Read the model definition and answer for the solid it produces. Units are mm, in the model's axes. A direction names the side the tool comes from. Give positions to 0.01 mm unless a question says otherwise; leave off trailing zeros. Write each loop counter-clockwise with the first axis right and the second up, starting at its lowest first coordinate (ties: lowest second). Pieces come first, ordered by that corner, then holes. Notation, with made-up numbers: M 41.25,73 L 93.25,73 A32 cw 93.25,110 Z; hole C -23.5,-1 d3. An arc over 180 degrees is marked long. Put each result on its own line as item: value.
from build123d import *

# Parameters (mm, degrees)
SKETCH_1_W          = 87.4
SKETCH_1_H          = 58
EXTRUDE_1_DEPTH     = 2
EXTRUDE_2_DEPTH     = 9
SKETCH_3_W          = 2
SKETCH_3_H          = 5
EXTRUDE_3_DEPTH     = 28
SKETCH_4_W          = 28
SKETCH_4_H          = 3
EXTRUDE_4_DEPTH     = 5.4
EXTRUDE_7_DEPTH     = 58
SKETCH_6_W          = 14.323261058
SKETCH_6_H          = 15
CUT_EXTRUDE_2_DEPTH = 58
SKETCH_8_W          = 87.4
SKETCH_8_H          = 14.7
CUT_EXTRUDE_3_DEPTH = 35
SKETCH_9_W          = 87.4
SKETCH_9_H          = 58
EXTRUDE_8_DEPTH     = 2
EXTRUDE_9_DEPTH     = 29
SKETCH_11_W         = 8.812157776
SKETCH_11_H         = 15
CUT_EXTRUDE_4_DEPTH = 13
SKETCH_13_W         = 87.4
SKETCH_13_H         = 0.5
CUT_EXTRUDE_6_DEPTH = 200


with BuildPart() as part:
    # 草图1 → 凸台-拉伸1 (new body)
    with BuildSketch(Plane.XY):
        Rectangle(SKETCH_1_W, SKETCH_1_H)
    extrude(amount=EXTRUDE_1_DEPTH)

    # 草图2 → 凸台-拉伸2 (add)
    with BuildSketch(Plane.XY.offset(2)):
        Polygon((-43.7, -25), (-43.7, -27), (-13.7, -27), (-13.7, 12.3), (-43.7, 12.3), (-43.7, 10.3), (-15.7, 10.3), (-15.7, -25), align=None)
    extrude(amount=EXTRUDE_2_DEPTH)

    # 草图3 → 凸台-拉伸3 (add)
    with BuildSketch(Plane.ZY.offset(15.7)):
        with Locations((10, 7.8)):
            Rectangle(SKETCH_3_W, SKETCH_3_H)
        with Locations((10, -22.5)):
            Rectangle(SKETCH_3_W, SKETCH_3_H)
    extrude(amount=EXTRUDE_3_DEPTH)

    # 草图4 → 凸台-拉伸4 (add)
    with BuildSketch(Plane.XY.offset(2)):
        with Locations((-29.7, 8.8)):
            Rectangle(SKETCH_4_W, SKETCH_4_H)
        with Locations((-29.7, -23.5)):
            Rectangle(SKETCH_4_W, SKETCH_4_H)
    extrude(amount=EXTRUDE_4_DEPTH)

    # 草图5 → 凸台-拉伸7 (add)
    with BuildSketch(Plane.XZ.offset(29)):
        Polygon((39.7, 2), (41.7, 4), (41.7, 2), align=None)
    extrude(amount=-EXTRUDE_7_DEPTH)

    # 草图6 → 切除-拉伸2 (cut)
    with BuildSketch(Plane.XY.offset(2)):
        with Locations((36.538369471, -21.5)):
            Rectangle(SKETCH_6_W, SKETCH_6_H)
        with Locations((36.538369471, 21.5)):
            Rectangle(SKETCH_6_W, SKETCH_6_H)
    extrude(amount=CUT_EXTRUDE_2_DEPTH, mode=Mode.SUBTRACT)

    # 草图8 → 切除-拉伸3 (cut)
    with BuildSketch(Plane.XY.offset(2)):
        with Locations((0, 21.65)):
            Rectangle(SKETCH_8_W, SKETCH_8_H)
    extrude(amount=-CUT_EXTRUDE_3_DEPTH, mode=Mode.SUBTRACT)

    # 草图9 → 凸台-拉伸8 (add)
    with BuildSketch(Plane(origin=(0, 0, 0), x_dir=(-1, 0, 0), z_dir=(0, 0, -1))):
        with Locations((0, -14.7)):
            Rectangle(SKETCH_9_W, SKETCH_9_H)
    extrude(amount=-EXTRUDE_8_DEPTH)

    # 草图10 → 凸台-拉伸9 (add)
    with BuildSketch(Plane.XZ.offset(14)):
        Polygon((41.7, 4), (41.7, 2), (39.7, 2), align=None)
    extrude(amount=EXTRUDE_9_DEPTH)

    # 草图11 → 切除-拉伸4 (cut)
    with BuildSketch(Plane.XY.offset(2)):
        with Locations((39.293921112, 6.8)):
            Rectangle(SKETCH_11_W, SKETCH_11_H)
        with Locations((39.293921112, -36.2)):
            Rectangle(SKETCH_11_W, SKETCH_11_H)
    extrude(amount=CUT_EXTRUDE_4_DEPTH, mode=Mode.SUBTRACT)

    # 草图13 → 切除-拉伸6 (cut)
    with BuildSketch(Plane(origin=(0, 14.3, 0), x_dir=(1, 0, 0), z_dir=(0, 1, 0))):
        with Locations((0, -0.25)):
            Rectangle(SKETCH_13_W, SKETCH_13_H)
    extrude(amount=-CUT_EXTRUDE_6_DEPTH, mode=Mode.SUBTRACT)


solid = part.part
(1) Section B-B on x = -34.5 is taken. Determine the outline of the cut face in (y, z), and give its area (3 significant figures).
Result:
outline: M -43.7,0.5 L 14.3,0.5 L 14.3,2 L 12.3,2 L 12.3,11 L 5.3,11 L 5.3,9 L 10.3,9 L 10.3,7.4 L 7.3,7.4 L 7.3,2 L -22,2 L -22,7.4 L -25,7.4 L -25,9 L -20,9 L -20,11 L -27,11 L -27,2 L -43.7,2 Z
area: 175 mm²
(2) Given pin 1 Ø1.8 at (x, z) = (-31.5, 8.5) entering from +Y; pin 2 Ø6 at (x, y) = (28.5, -30) entering from +Z; pin 3 Ø1 at (x, z) = (-35, 10.5) entering from -Y, each flat-ended and moving along its own axis, determine where each tip first touches the part or whether it passes through.
Result:
pin 1: stops at y = 12.3
pin 2: stops at z = 2
pin 3: stops at y = -27
(3) Section C-C on z = 6.25 is taken. Determine the outline of the cut face in (x, y).
Result:
outline: M -43.7,-27 L -13.7,-27 L -13.7,12.3 L -43.7,12.3 L -43.7,7.3 L -15.7,7.3 L -15.7,-22 L -43.7,-22 Z
(4) Section A-A on y = -16.5 is taken. Determine the outline of the cut face in (x, z), and give its area (3 significant figures).
Result:
outline: M -43.7,0.5 L 43.7,0.5 L 43.7,2 L 41.7,2 L 41.7,4 L 39.7,2 L -13.7,2 L -13.7,11 L -15.7,11 L -15.7,2 L -43.7,2 Z
area: 151 mm²
(5) Section D-D on y = 9 is taken. Determine the outline of the cut face in (x, z).
Result:
outline: M -43.7,0.5 L 43.7,0.5 L 43.7,2 L -13.7,2 L -13.7,11 L -43.7,11 L -43.7,9 L -15.7,9 L -15.7,7.4 L -43.7,7.4 Z
(6) For a pull along X with two mould halves and no side action, classify faces 1 (the face through (-43.7, -12.7, 1.8)), 2 (the face through (10, -14, 2)), 3 (the face through (41.7, -15, 3)), 4 (the face through (-15, -8, 11)) as +X half, -X half, draft (parallel to the pull), parting line (faces both ways), or undercut.
Result:
face 1: -X half
face 2: undercut
face 3: +X half
face 4: draft
(7) Which of the six approach directions +Z, -Z, +X, -X, +Y, -Y give full straight-line access (tool end or side, diameter ignored) to faces 5 (the face through (-28, 12.3, 6)), 6 (the face through (-29, -27, 6)), 7 (the face through (-30, -25, 8))?
Result:
face 5: +Z, +X, -X, +Y
face 6: +Z, -X, -Y
face 7: -X
(8) Straight lines are drawn through the part: line 1 along Y through (x, z) = (-19.5, 8.5); line 2 along X through (y, z) = (-4.5, 10.5); line 3 along Z through (x, y) = (-19.5, -9.5). For each, find the intervals that lie inside material, in ascending order. Write a range as from..to.
Result:
line 1: y = -27..-25, 10.3..12.3
line 2: x = -15.7..-13.7
line 3: z = 0.5..2
